Build history of the part. All positions in model axes, mm. A direction names the side the tool comes from. Give positions to 0.01 mm unless a question says otherwise; leave off trailing zeros. Loops run counter-clockwise (first coordinate to the right, second up) from the corner with the lowest first, then second, coordinate; pieces in that order, holes last. Notation, with made-up numbers: M 75.25,23.25 L 86.25,23.25 A29 ccw 86.25,51.25 Z; hole C 80,89 d5. An arc over 180 degrees is marked long. Put each result on its own line as item: value.
```python
from build123d import *

# Parameters (mm, degrees)
SKETCH1_W           = 4
SKETCH1_H           = 5
BOSS_EXTRUDE1_DEPTH = 2
SKETCH2_W           = 4
SKETCH2_H           = 2
BOSS_EXTRUDE2_DEPTH = 2
BOSS_EXTRUDE3_DEPTH = 2


with BuildPart() as part:
    # Sketch1 → Boss-Extrude1 (new body)
    with BuildSketch(Plane.XY):
        Rectangle(SKETCH1_W, SKETCH1_H)
    extrude(amount=BOSS_EXTRUDE1_DEPTH)

    # Sketch2 → Boss-Extrude2 (add)
    with BuildSketch(Plane.XY.offset(2)):
        with Locations((0, -1.5)):
            Rectangle(SKETCH2_W, SKETCH2_H)
    extrude(amount=BOSS_EXTRUDE2_DEPTH)

    # Sketch3 → Boss-Extrude3 (add)
    with BuildSketch(Plane(origin=(0, -0.5, 0), x_dir=(1, 0, 0), z_dir=(0, 1, 0))):
        Polygon((2, -4), (4, -2), (2, -2), align=None)
    extrude(amount=-BOSS_EXTRUDE3_DEPTH)


solid = part.part
```
Q1. Slice it at C-C (z = 2.35). List the corners of the cut face in (x, y), and give its area (3 significant figures).
Here are the results:
outline: M -2,-2.5 L 3.65,-2.5 L 3.65,-0.5 L -2,-0.5 Z
area: 11.3 mm²
Q2. Slice it at D-D (y = 0.9). List the corners of the cut face in (x, z), and give its area (3 significant figures).
Here are the results:
outline: M -2,0 L 2,0 L 2,2 L -2,2 Z
area: 8.00 mm²
Q3. Probe line 1 (X direction, y = -0.85, z = 0.35); line 2 (Y direction, x = 1.4, z = 3.4); line 3 (Z direction, x = 0.9, y = 2.2). List the from-to ranges inside material, lowest first. Write a range as from..to.
Here are the results:
line 1: -2..2
line 2: -2.5..-0.5
line 3: 0..2
Q4. Tool access for faces 1 (the flat face through (0, 1, 2)), 2 (the flat face through (3, -1, 2)), 3 (the flat face through (-2, -1, 2)): list every direction of +Z, -Z, +X, -X, +Y, -Y with a clear straight run to the whole face (end or side of a thin tool).
Here are the results:
face 1: +Z, +X, -X, +Y
face 2: -Z, +X, +Y, -Y
face 3: +Z, -Z, -X, +Y, -Y
Q5. Slice it at A-A (x = 0.25). List the corners of the cut face in (y, z).
Here are the results:
outline: M -2.5,0 L 2.5,0 L 2.5,2 L -0.5,2 L -0.5,4 L -2.5,4 Z
Q6. Slice it at B-B (y = -0.8). List the corners of the cut face in (x, z), and give its area (3 significant figures).
Here are the results:
outline: M -2,0 L 2,0 L 2,2 L 4,2 L 2,4 L -2,4 Z
area: 18.0 mm²
Q7. Drop flat-ended pins along their axis: pin 1 Ø1.6 at (x, z) = (-0.5, 2.5) entering from +Y; pin 2 Ø2 at (x, y) = (3.5, -2) entering from -Z; pin 3 Ø2.5 at (x, y) = (0.5, 1.5) entering from +Z; pin 4 Ø1.5 at (y, z) = (2, 0.5) entering from +X. Give the stop position or say it passes through.
Here are the results:
pin 1: y = 2.5
pin 2: z = 2
pin 3: z = 2
pin 4: x = 2
